```python
from build123d import *

# Parameters (mm, degrees)
SKETCH1_R           = 5
SKETCH1_R_2         = 1.6
BOSS_EXTRUDE1_DEPTH = 3
SKETCH2_R           = 4
CUT_EXTRUDE1_DEPTH  = 2.5
CHAMFER1_SIZE       = 0.2
FILLET2_R           = 0.2


with BuildPart() as part:
    # Sketch1 → Boss-Extrude1 (new body)
    with BuildSketch(Plane(origin=(0, 0, 0), x_dir=(1, 0, 0), z_dir=(0, 1, 0))):
        with Locations(Location((0, 0, 0), (0, 0, 270))):
            Circle(SKETCH1_R)
        with Locations(Location((0, 0, 0), (0, 0, 270))):
            Circle(SKETCH1_R_2, mode=Mode.SUBTRACT)
    extrude(amount=BOSS_EXTRUDE1_DEPTH)

    # Sketch2 → Cut-Extrude1 (cut)
    with BuildSketch(Plane(origin=(0, 3, 0), x_dir=(1, 0, 0), z_dir=(0, 1, 0))):
        with Locations(Location((0, 0, 0), (0, 0, 270))):
            Circle(SKETCH2_R)
    extrude(amount=-CUT_EXTRUDE1_DEPTH, mode=Mode.SUBTRACT)

    # Chamfer1
    chamfer1_edges = [part.edges().sort_by_distance(p)[0] for p in [
        (0, 3, -4),
    ]]
    chamfer(chamfer1_edges, length=CHAMFER1_SIZE)

    # Fillet2
    fillet2_edges = [part.edges().sort_by_distance(p)[0] for p in [
        (0, 3, -4.2),
        (0, 0, -5),
        (0, 3, -5),
    ]]
    fillet(fillet2_edges, radius=FILLET2_R)


solid = part.part
```
Geometry check sheet. Reference: the model listing, model coordinates, mm. Give positions to 0.01 mm unless a question says otherwise; leave off trailing zeros. Order: outer loops, then holes, each group sorted by start corner. A loop starts at its lowest first (then second) coordinate and runs counter-clockwise, first axis right, second up. Notation, with made-up numbers: (71, 8) - (129, 8) arc R30 cw to (129, 41) - close; hole circle Ø2 at (-0.5, 25). An arc over 180 degrees is marked (long way). Write item = value, one per line. Start each with the question number.
1) Gauge pin test, flat ends, axial feed: pin 1 Ø1 at (x, z) = (1.5, -1.5) entering from -Y; pin 2 Ø2.5 at (x, z) = (-1.5, 0.5) entering from +Y. Record the tip position at first contact, or that the pin passes through.
2) Draft check along Z on faces 1 (the flat face through (2, 3, -4)), 2 (the cylindrical face through (-3.905, 1.666, -0.867)), 3 (the flat face through (0, 0.5, 2)), 4 (the cylindrical face through (-4.88, 1.48, -1.08)). Enter one of: released by +Z, released by -Z, zero draft, split by the parting line, or undercut.
3) Scan lines: L1, parallel to X at y = 0.35, z = 0; L2, parallel to X at y = 1.2, z = 0; L3, parallel to Z at x = 1.5, y = 2.45. Record each from-to range of solid material in increasing order.
4) Section check A-A (z = 0). Enter the section's corners in (x, y), then the cut area to 3 significant figures.
5) Section check B-B (y = 2.45). Enter the section's corners in (x, z).
Geometry check:
q1.pin_1 = 0
q1.pin_2 = 0.5
q2.face_1 = zero draft
q2.face_2 = undercut
q2.face_3 = undercut
q2.face_4 = split by the parting line
q3.L1 = -5 to -1.6, 1.6 to 5
q3.L2 = -5 to -4, 4 to 5
q3.L3 = -4.77 to -3.71, 3.71 to 4.77
q4.outline = (-5, 0.2) arc R0.2 ccw to (-4.8, 0) - (-1.6, 0) - (-1.6, 0.5) - (-4, 0.5) - (-4, 2.8) - (-4.14, 2.94) arc R0.2 ccw to (-4.28, 3) - (-4.8, 3) arc R0.2 ccw to (-5, 2.8) - close; (1.6, 0) - (4.8, 0) arc R0.2 ccw to (5, 0.2) - (5, 2.8) arc R0.2 ccw to (4.8, 3) - (4.28, 3) arc R0.2 ccw to (4.14, 2.94) - (4, 2.8) - (4, 0.5) - (1.6, 0.5) - close
q4.area = 8.32 mm2
q5.outline = circle Ø10 at (0, 0); hole circle Ø8 at (0, 0)
